Work out the finished part from the listing and answer in its coordinate system (mm). A direction names the side the tool comes from. Give positions to 0.01 mm unless a question says otherwise; leave off trailing zeros. Write each loop counter-clockwise with the first axis right and the second up, starting at its lowest first coordinate (ties: lowest second). Pieces come first, ordered by that corner, then holes. Notation, with made-up numbers: (48, 23) -> (60, 23) arc R10 cw to (60, 29) -> close; hole circle Ø6 at (53.5, 87). An arc over 180 degrees is marked (long way). Use a Markdown table: item, result. Add a question column.
Q1. Section C-C, the plane z = 9 is taken. Give the vertices of the cut face in (x, y).
Q2. Consider line 1 (Z direction, x = 36.5, y = -2.5); line 2 (Z direction, x = 20.5, y = -16.25); line 3 (X direction, y = -2.5, z = 21). Determine where each line is inside the solid, lowest interval first.
Q3. For a pull along X with two mould halves and no side action, classify faces 1 (the face through (45.43, -1.52, 11.9)), 2 (the face through (20, -28, 2)), 3 (the face through (1.99, -15.32, 28.86)) as pulls with the +X half, pulls with the -X half, needs draft (parallel to the pull), parting line crosses it, or undercut.
Q4. Section D-D, the plane z = 32.5 is taken. Give the vertices of the cut face in (x, y), plus the area to 3 significant figures.
Q5. Section B-B, the plane x = -15 is taken. Give the vertices of the cut face in (y, z), plus the area to 3 significant figures.
Q6. For faces 4 (the face through (-7.1, -15.3, 44.4)), 5 (the face through (-0.54, -1.52, 13.08)), 6 (the face through (42, -15, 16)), 7 (the face through (-6.724, -15.325, 19.147)), 8 (the face through (-19.72, -15.32, 41.66)), determine the directions among +Z, -Z, +X, -X, +Y, -Y from which every point of the face is accessible in a straight line to the end or side of a thin tool.
Q7. Each of these flat-tipped pins is pushed along its axis until it touches: pin 1 Ø6 at (x, y) = (41.5, -17.5) entering from +Z; pin 2 Ø2 at (y, z) = (-14, 40) entering from +X; pin 3 Ø3 at (y, z) = (-18, 17) entering from -X; pin 4 Ø3 at (y, z) = (-9, 10.5) entering from +X. Where does it stop, or does it pass through?
Q8. Section A-A, the plane y = -13.75 is taken. State how many separate pieces and enclosed holes the cut face has, plus the area to 3 significant figures.
from build123d import *

# Parameters (mm, degrees)
F1_DEPTH = 3
F2_W     = 8
F2_H     = 3.75
F3_DEPTH = 25
F4_R     = 3
F5_DEPTH = 3.001


with BuildPart() as f1:
    # F0 (on Front) → F1 (new body)
    with BuildSketch(Plane.XZ):
        Polygon((-25, 43.30127), (0, 0), (50, 0), (50, 18), (10.392305, 18), (-9.411543, 52.30127), align=None)
    extrude(amount=F1_DEPTH)

    # F2 (on face) → F3 (join)
    with BuildSketch(Plane.XZ.offset(3)):
        with Locations((46, 16.125)):
            Rectangle(F2_W, F2_H)
        with Locations((46, 1.875)):
            Rectangle(F2_W, F2_H)
        with Locations((20, 1.875)):
            Rectangle(F2_W, F2_H)
        with Locations((20, 16.125)):
            Rectangle(F2_W, F2_H)
        Polygon((4.340862, 20.981406), (7.588457, 22.856406), (3.588457, 29.78461), (0.340862, 27.90961), align=None)
        Polygon((-12, 20.78461), (-8, 13.856406), (-4.752405, 15.731406), (-8.752405, 22.65961), align=None)
        Polygon((-17.752405, 38.248067), (-21.752405, 45.17627), (-25, 43.30127), (-21, 36.373067), align=None)
        Polygon((-8.659138, 43.498067), (-5.411543, 45.373067), (-9.411543, 52.30127), (-12.659138, 50.42627), align=None)
    extrude(amount=F3_DEPTH)

    # F4 (on face) → F5 (cut, through all)
    with BuildSketch(Plane.XZ.offset(3)):
        with BuildLine():
            ThreePointArc((3.593267, 14.776279), (4.525118, 15.990692), (4.325318, 17.50833))
            Line((4.325318, 17.50833), (-11.174682, 44.355118))
            ThreePointArc((-11.174682, 44.355118), (-12.389095, 45.286969), (-13.906733, 45.087169))
            Line((-13.906733, 45.087169), (-16.504809, 43.587169))
            ThreePointArc((-16.504809, 43.587169), (-17.436661, 42.372756), (-17.23686, 40.855118))
            Line((-17.23686, 40.855118), (-1.73686, 14.00833))
            ThreePointArc((-1.73686, 14.00833), (-0.522448, 13.076479), (0.995191, 13.276279))
            Line((0.995191, 13.276279), (3.593267, 14.776279))
        make_face()
        with BuildLine():
            Line((44, 12.5), (13, 12.5))
            ThreePointArc((13, 12.5), (11.585786, 11.914214), (11, 10.5))
            Line((11, 10.5), (11, 7.5))
            ThreePointArc((11, 7.5), (11.585786, 6.085786), (13, 5.5))
            Line((13, 5.5), (44, 5.5))
            ThreePointArc((44, 5.5), (45.414214, 6.085786), (46, 7.5))
            Line((46, 7.5), (46, 10.5))
            ThreePointArc((46, 10.5), (45.414214, 11.914214), (44, 12.5))
        make_face()
        with Locations((5.196152, 9)):
            Circle(F4_R)
    extrude(amount=-F5_DEPTH, mode=Mode.SUBTRACT)


solid = f1.part
Result set:
| question | item | result |
|---|---|---|
| 1 | outline | (-5.2, -3) -> (2.2, -3) -> (2.2, 0) -> (-5.2, 0) -> close; (8.2, -3) -> (11, -3) -> (11, 0) -> (8.2, 0) -> close; (46, -3) -> (50, -3) -> (50, 0) -> (46, 0) -> close |
| 2 | line 1 | z = 0 to 5.5, 12.5 to 18 |
| 2 | line 2 | z = 0 to 3.75, 14.25 to 18 |
| 2 | line 3 | x = -12.12 to -5.77, 2.31 to 8.66 |
| 3 | face 1 | undercut |
| 3 | face 2 | needs draft |
| 3 | face 3 | pulls with the -X half |
| 4 | outline | (-18.76, -3) -> (-12.41, -3) -> (-12.41, 0) -> (-18.76, 0) -> close; (-4.33, -3) -> (2.02, -3) -> (2.02, 0) -> (-4.33, 0) -> close |
| 4 | area | 38.1 mm2 |
| 5 | outline | (-3, 25.98) -> (0, 25.98) -> (0, 36.98) -> (-3, 36.98) -> close; (-3, 44.46) -> (0, 44.46) -> (0, 49.07) -> (-3, 49.07) -> close |
| 5 | area | 46.9 mm2 |
| 6 | face 4 | +X, -Y |
| 6 | face 5 | +Y, -Y |
| 6 | face 6 | +Z, -Z, -Y |
| 6 | face 7 | -Y |
| 6 | face 8 | +Z, -Y |
| 7 | pin 1 | stops at z = 18 |
| 7 | pin 2 | stops at x = -18.19 |
| 7 | pin 3 | stops at x = -10.68 |
| 7 | pin 4 | passes through |
| 8 | separate pieces | 8 |
| 8 | enclosed holes | 0 |
| 8 | area | 240 mm2 |
